CAD build for the part. Positions are in the model's coordinates, mm. Face numbers are marked on the shaded views. A direction names the side the tool comes from. Coordinates: 2 decimals unless noted, no trailing zeros. Loops run counter-clockwise (first coordinate to the right, second up) from the corner with the lowest first, then second, coordinate; pieces in that order, holes last. Notation, with made-up numbers: (-35, -24.75) -> (-10, -24.75) arc R12 cw to (-10, -18.75) -> close; hole circle Ø2 at (64, 6). An arc over 180 degrees is marked (long way). Answer as CSV lines item,"result". Start each with the question number.
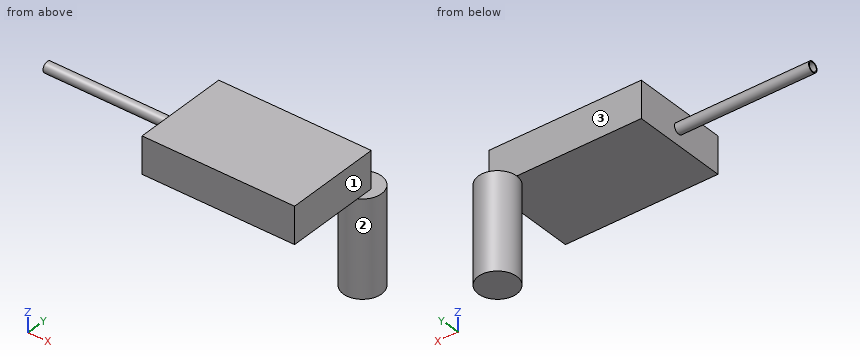
from build123d import *

# Parameters (mm, degrees)
F0_W     = 40.230050683
F0_H     = 9.7180828452
F1_DEPTH = 25.4
F2_R     = 1.3894743623
F2_R_2   = 1.1592895912
F3_DEPTH = 35.3568
F4_R     = 5.0629514974
F5_DEPTH = 25.4


with BuildPart() as f1:
    # F0 (on Front) → F1 (new body)
    with BuildSketch(Plane.XZ):
        with Locations((-104.2651683092, 49.1601750255)):
            Rectangle(F0_W, F0_H)
    extrude(amount=F1_DEPTH)

    # F2 (on face) → F3 (join)
    with BuildSketch(Plane(origin=(-124.3801936507, 0, 0), x_dir=(0, -1, 0), z_dir=(-1, 0, 0))):
        with Locations((12.4141043052, 48.6199855804)):
            Circle(F2_R)
        with Locations((12.4141043052, 48.6199855804)):
            Circle(F2_R_2, mode=Mode.SUBTRACT)
    extrude(amount=F3_DEPTH)

    # F4 (on face) → F5 (join)
    with BuildSketch(Plane(origin=(0, 0, 44.3011336029), x_dir=(1, 0, 0), z_dir=(0, 0, -1))):
        with Locations((-86.4652916789, 0)):
            Circle(F4_R)
    extrude(amount=F5_DEPTH)


solid = f1.part
Item 1: Flat gauge pins, fed straight in: pin 1 Ø12 at (y, z) = (-16, 45.5) entering from +X; pin 2 Ø8 at (x, y) = (-141.5, -12) entering from -Z; pin 3 Ø0.7 at (y, z) = (-12.5, 48.5) entering from -X; pin 4 Ø2.5 at (y, z) = (-12.41, 48.62) entering from -X. Where does each tip first touch, or does it go through?
Item 2: Wall check: probe 1 along Z at (x, y) = (-152.5, -11.5); probe 2 along X at (y, z) = (-24, 49.5); probe 3 along Z at (x, y) = (-120.5, -1.5). Give the ranges that are in metal, low to high.
Item 3: Saw through at B-B (z = 28.5). Write the cut outline in (x, y).
Item 4: Saw through at C-C (y = 1). Write the cut outline in (x, z).
Item 5: Which spindle directions (+Z, -Z, +X, -X, +Y, -Y) get a long thin tool onto all of the face, cutting with end or side? Do the marked faces 1, 2 and 3. Say none if no direction does.
Item 6: Saw through at A-A (x = -114.5). Write the cut outline in (y, z), plus the area to 3 significant figures.
Geometry check:
1,pin 1,"x = -84.15"
1,pin 2,"z = 47.23"
1,pin 3,"x = -124.38"
1,pin 4,"x = -159.74"
2,probe 1,"47.57 to 47.91, 49.33 to 49.67"
2,probe 2,"-124.38 to -84.15"
2,probe 3,"44.3 to 54.02"
3,outline,"circle Ø10.13 at (-86.47, 0)"
4,outline,"(-91.43, 18.9) -> (-81.5, 18.9) -> (-81.5, 44.3) -> (-91.43, 44.3) -> close"
5,face 1,"+Z, +X, +Y, -Y"
5,face 2,"-Z"
5,face 3,"+Z, +X, -X, +Y"
6,outline,"(-25.4, 44.3) -> (0, 44.3) -> (0, 54.02) -> (-25.4, 54.02) -> close"
6,area,"247 mm2"
